Part print with two shaded views. Sizes in mm from the minimum x, y, z corner. Round coordinates to 2 decimals unless told otherwise and drop trailing zeros. Order: outer loops, then holes, each group sorted by start corner. A loop starts at its lowest first (then second) coordinate and runs counter-clockwise, first axis right, second up. Notation, with made-up numbers: M 17,26.25 L 61,26.25 A14 cw 61,37.25 Z; hole C 66.5,23.25 d1. An arc over 180 degrees is marked long. Answer as a JSON object with one key per item and string values.
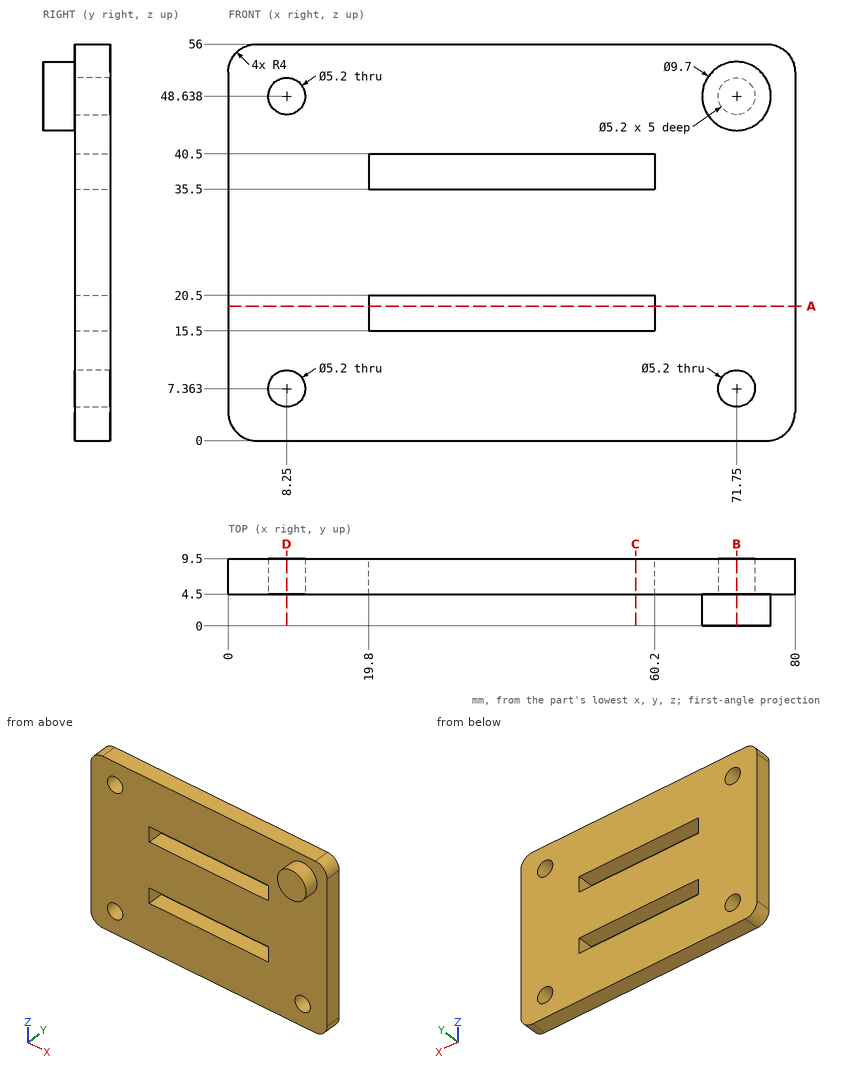
Item 1: Saw through at D-D on x = 8.25. List the corners of the cut face in (y, z), and give its area (3 significant figures).
Worked answers:
{"outline": "M 4.5,0 L 9.5,0 L 9.5,4.76 L 4.5,4.76 Z; M 4.5,9.96 L 9.5,9.96 L 9.5,46.04 L 4.5,46.04 Z; M 4.5,51.24 L 9.5,51.24 L 9.5,56 L 4.5,56 Z", "area": "228 mm2"}
Item 2: Wall check: line 1 along Z through (x, y) = (25, 7); line 2 along Z through (x, y) = (71.75, 6.1); line 3 along X through (y, z) = (6.5, 38). Give the ranges that are in metal, low to high. Write a range as [from, to].
Worked answers:
{"line 1": "z = [0, 15.5], [20.5, 35.5], [40.5, 56]", "line 2": "z = [0, 4.76], [9.96, 46.04], [51.24, 56]", "line 3": "x = [0, 19.8], [60.2, 80]"}
Item 3: Saw through at C-C on x = 57.5. List the corners of the cut face in (y, z).
Worked answers:
{"outline": "M 4.5,0 L 9.5,0 L 9.5,15.5 L 4.5,15.5 Z; M 4.5,20.5 L 9.5,20.5 L 9.5,35.5 L 4.5,35.5 Z; M 4.5,40.5 L 9.5,40.5 L 9.5,56 L 4.5,56 Z"}
Item 4: Saw through at B-B on x = 71.75. List the corners of the cut face in (y, z), and give its area (3 significant figures).
Worked answers:
{"outline": "M 0,43.79 L 4.5,43.79 L 4.5,9.96 L 9.5,9.96 L 9.5,46.04 L 4.5,46.04 L 4.5,51.24 L 9.5,51.24 L 9.5,56 L 4.5,56 L 4.5,53.49 L 0,53.49 Z; M 4.5,0 L 9.5,0 L 9.5,4.76 L 4.5,4.76 Z", "area": "272 mm2"}
Item 5: Drop flat-ended pins along their axis: pin 1 Ø2.5 at (x, z) = (71.5, 48) entering from +Y; pin 2 Ø8.5 at (x, z) = (8.25, 48.64) entering from -Y. Give the stop position or say it passes through.
Worked answers:
{"pin 1": "stops at y = 4.5", "pin 2": "stops at y = 4.5"}
Item 6: Saw through at A-A on z = 19. List the corners of the cut face in (x, y), and give its area (3 significant figures).
Worked answers:
{"outline": "M 0,4.5 L 19.8,4.5 L 19.8,9.5 L 0,9.5 Z; M 60.2,4.5 L 80,4.5 L 80,9.5 L 60.2,9.5 Z", "area": "198 mm2"}
